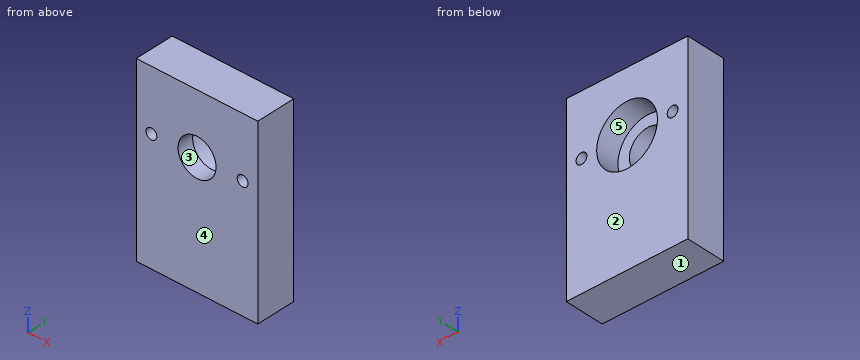
```python
from build123d import *

# Parameters (mm, degrees)
F0_W     = 25.4
F0_H     = 38.1
F0_R     = 6.35
F0_R_2   = 3.96875
F1_DEPTH = 8.255
F2_DEPTH = 4.8895
F3_D     = 2.2606


with BuildPart() as f1:
    # F0 (on Front) → F1 (new body)
    with BuildSketch(Plane.XZ):
        with Locations((12.7, 19.05)):
            Rectangle(F0_W, F0_H)
        with Locations((12.7, 25.4)):
            Circle(F0_R, mode=Mode.SUBTRACT)
        with Locations((12.7, 25.4)):
            Circle(F0_R)
        with Locations((12.7, 25.4)):
            Circle(F0_R_2, mode=Mode.SUBTRACT)
    extrude(amount=F1_DEPTH)

    # F0 (on Front) → F2 (cut)
    with BuildSketch(Plane.XZ):
        with Locations((12.7, 25.4)):
            Circle(F0_R)
        with Locations((12.7, 25.4)):
            Circle(F0_R_2, mode=Mode.SUBTRACT)
    extrude(amount=F2_DEPTH, mode=Mode.SUBTRACT)

    # F3 (through all)
    with Locations(Plane(origin=(0, 0, 0), x_dir=(1, 0, 0), z_dir=(0, 1, 0))):
        with Locations((22.225, -25.4), (3.175, -25.4)):
            Hole(F3_D / 2)


solid = f1.part
```
Part model, mm, in its own coordinate system. Face numbers are marked on the shaded views. A direction names the side the tool comes from. Coordinates: 2 decimals unless noted, no trailing zeros. Order: outer loops, then holes, each group sorted by start corner. A loop starts at its lowest first (then second) coordinate and runs counter-clockwise, first axis right, second up. Notation, with made-up numbers: (88.25, -3.75) - (95.25, -3.75) arc R37 cw to (95.25, 32.25) - close; hole circle Ø9 at (-7.5, 37.25). An arc over 180 degrees is marked (long way). Return JSON: item names as keys, results as strings. Group by question number.
Item 1: Cut at A-A (z = 25.4). State how many separate pieces and enclosed holes the cut face has, plus the area to 3 significant figures.
Item 2: Which spindle directions (+Z, -Z, +X, -X, +Y, -Y) get a long thin tool onto all of the face, cutting with end or side? Do the marked faces 4 and 5. Say none if no direction does.
Item 3: Pin check, flat tip, straight feed: pin 1 (6.5 mm diameter, centred on x = 14.5, z = 28, fed in from +Y). Stop position of the tip, or through.
Item 4: Pull direction Z, two halves, no side cores. Call the marked faces 1, 2 and 3: pulls with the +Z half, pulls with the -Z half, needs draft (parallel to the pull), parting line crosses it, or undercut.
Item 5: Cut at D-D (x = 2.75). List the corners of the cut face in (y, z) (3 decimals).
Item 6: Drill centre lines: probe 1 along Z at (x, y) = (12.7, -3.25); probe 2 along X at (y, z) = (-7, 25); probe 3 along Z at (x, y) = (12.7, -6.1). Where is each one in solid material? Low to high. Write a range as from..to.
Item 7: Cut at C-C (y = -7.5). List the corners of the cut face in (x, z) (1 decimal).
Check values:
{
 "1": {"separate pieces": "4", "enclosed holes": "0", "area": "83.5 mm2"},
 "2": {"face 4": "+Z, -Z, +X, -X, -Y", "face 5": "+Y"},
 "3": {"pin 1": "stops at y = 0"},
 "4": {"face 1": "pulls with the -Z half", "face 2": "needs draft", "face 3": "undercut"},
 "5": {"outline": "(-8.255, 0) - (0, 0) - (0, 24.353) - (-8.255, 24.353) - close; (-8.255, 26.447) - (0, 26.447) - (0, 38.1) - (-8.255, 38.1) - close"},
 "6": {"probe 1": "z = 0..19.05, 31.75..38.1", "probe 2": "x = 0..2.12, 4.23..8.75, 16.65..21.17, 23.28..25.4", "probe 3": "z = 0..21.43, 29.37..38.1"},
 "7": {"outline": "(0, 0) - (25.4, 0) - (25.4, 38.1) - (0, 38.1) - close; hole circle Ø2.3 at (3.2, 25.4); hole circle Ø7.9 at (12.7, 25.4); hole circle Ø2.3 at (22.2, 25.4)"}
}
